Geometry: final body of the model. Coordinates: model frame, mm. Round coordinates to 2 decimals unless told otherwise and drop trailing zeros. Write each loop counter-clockwise with the first axis right and the second up, starting at its lowest first coordinate (ties: lowest second). Pieces come first, ordered by that corner, then holes. Notation, with made-up numbers: M 41,46 L 81,46 A25 cw 81,81 Z; hole C -8.5,-1.75 d9. An arc over 180 degrees is marked long. Use one line per item in the form item = value. Start each with the question number.
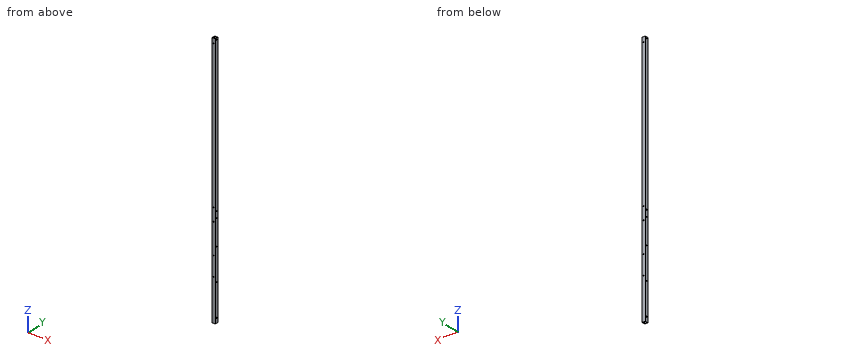
from build123d import *

# Parameters (mm, degrees)
SKETCH_1_W             = 10
SKETCH_1_H             = 10
SKETCH_1_W_2           = 8
SKETCH_1_H_2           = 8
EXTRUDE_1_DEPTH        = 800
SKETCH_3_R             = 1.6
CUT_EXTRUDE_2_DEPTH    = 801.078121186
SKETCH_4_R             = 1.6
CUT_EXTRUDE_3_DEPTH    = 801.078121186
SKETCH_5_R             = 1.6
CUT_EXTRUDE_4_DEPTH    = 801.078121186
PATTERN_LINEAR_1_COUNT = 4
PATTERN_LINEAR_1_PITCH = 100


with BuildPart() as part:
    # ｽｹｯﾁ1 → ﾎﾞｽ - 押し出し1 (new body)
    with BuildSketch(Plane.XY):
        Rectangle(SKETCH_1_W, SKETCH_1_H)
        Rectangle(SKETCH_1_W_2, SKETCH_1_H_2, mode=Mode.SUBTRACT)
    extrude(amount=EXTRUDE_1_DEPTH)

    # ｽｹｯﾁ3 → ｶｯﾄ - 押し出し2 (cut, through all)
    with BuildSketch(Plane(origin=(0, 5, 0), x_dir=(1, 0, 0), z_dir=(0, 1, 0))):
        with Locations(Location((0, -785, 0), (0, 0, 270))):
            Circle(SKETCH_3_R)
        with Locations(Location((0, -190, 0), (0, 0, 270))):
            Circle(SKETCH_3_R)
        with Locations(Location((0, -130, 0), (0, 0, 270))):
            Circle(SKETCH_3_R)
        with Locations(Location((0, -325, 0), (0, 0, 270))):
            Circle(SKETCH_3_R)
        with Locations(Location((0, -285, 0), (0, 0, 270))):
            Circle(SKETCH_3_R)
    extrude(amount=-CUT_EXTRUDE_2_DEPTH, mode=Mode.SUBTRACT)

    # ｽｹｯﾁ4 → ｶｯﾄ - 押し出し3 (cut, through all)
    with BuildSketch(Plane.ZY.offset(5)):
        with Locations((795, 0)):
            Circle(SKETCH_4_R)
        with Locations((295, 0)):
            Circle(SKETCH_4_R)
    extrude(amount=-CUT_EXTRUDE_3_DEPTH, mode=Mode.SUBTRACT)

    # ｽｹｯﾁ5 → ｶｯﾄ - 押し出し4 (cut, through all)
    with BuildSketch(Plane(origin=(5, 0, 0), x_dir=(0, 0, -1), z_dir=(1, 0, 0))):
        with Locations((-15, 0)):
            Circle(SKETCH_5_R)
    cut_extrude_4 = extrude(amount=-CUT_EXTRUDE_4_DEPTH, mode=Mode.SUBTRACT)

    # 直線ﾊﾟﾀｰﾝ1: ｶｯﾄ - 押し出し4 ×4
    with Locations(*[(0, 0, i * PATTERN_LINEAR_1_PITCH) for i in range(1, PATTERN_LINEAR_1_COUNT)]):
        add(cut_extrude_4, mode=Mode.SUBTRACT)


solid = part.part
1. Contact query for a flat-ended pin moving along its axis: pin 1 (2.5 mm diameter, centred on x = 0, z = 285, fed in from +Y). Output: stop coordinate, or through.
2. Ray query, probe 1 along X at (y, z) = (3.75, 469.5); probe 2 along X at (y, z) = (-4.4, 190). Return the intervals inside material, ascending.
3. Section query B-B (y = 0). Give the number of separate pieces and of enclosed holes in the cut face, then the cut area to 3 significant figures.
4. Section query A-A (z = 622). Return loops of the section in (x, y).
Checks:
q1.pin_1 = through
q2.probe_1 = -5 to -4, 4 to 5
q2.probe_2 = -5 to -1.6, 1.6 to 5
q3.separate_pieces = 14
q3.enclosed_holes = 0
q3.area = 1,560 mm^2
q4.outline = M -5,-5 L 5,-5 L 5,5 L -5,5 Z; hole M -4,-4 L 4,-4 L 4,4 L -4,4 Z
